```python
from build123d import *

# Parameters (mm, degrees)
SKETCH_1_W          = 76
SKETCH_1_H          = 60
EXTRUDE_1_DEPTH     = 2
EXTRUDE_2_DEPTH     = 3.35
SKETCH_2_W          = 76
SKETCH_2_H          = 60
CUT_EXTRUDE_1_DEPTH = 2.95
SKETCH_3_R          = 1.715
CUT_EXTRUDE_2_DEPTH = 10
SKETCH_5_R          = 1.5
CUT_EXTRUDE_3_DEPTH = 45.193605611
SKETCH_6_R          = 2.5
CUT_EXTRUDE_4_DEPTH = 45.111815616
CUT_EXTRUDE_5_DEPTH = 4
CUT_EXTRUDE_6_DEPTH = 4
CUT_EXTRUDE_7_DEPTH = 4


with BuildPart() as part:
    # 草圖1 → 填料-伸長1 (new body)
    with BuildSketch(Plane.XY):
        Rectangle(SKETCH_1_W, SKETCH_1_H)
        with BuildLine():
            Line((-6.042909564, -9.905650781), (-7.592909564, -12.590329533))
            ThreePointArc((-7.592909564, -12.590329533), (-7.896512744, -12.823292446), (-8.275922266, -12.773342235))
            Line((-8.275922266, -12.773342235), (-10.007973074, -11.773342235))
            ThreePointArc((-10.007973074, -11.773342235), (-10.240935987, -11.469739056), (-10.190985776, -11.090329533))
            Line((-10.190985776, -11.090329533), (-8.640985776, -8.405650781))
            ThreePointArc((-8.640985776, -8.405650781), (-8.337382596, -8.172687868), (-7.957973074, -8.22263808))
            Line((-7.957973074, -8.22263808), (-6.225922266, -9.22263808))
            ThreePointArc((-6.225922266, -9.22263808), (-5.992959353, -9.526241259), (-6.042909564, -9.905650781))
        make_face(mode=Mode.SUBTRACT)
        with BuildLine():
            ThreePointArc((-14.313100093, -9.230040965), (-14.996112795, -9.413053667), (-15.179125497, -8.730040965))
            Line((-15.179125497, -8.730040965), (-13.179125497, -5.26593935))
            ThreePointArc((-13.179125497, -5.26593935), (-12.496112795, -5.082926648), (-12.313100093, -5.76593935))
            Line((-12.313100093, -5.76593935), (-14.313100093, -9.230040965))
        make_face(mode=Mode.SUBTRACT)
        with BuildLine():
            ThreePointArc((11.146484837, -8.780487805), (10.646484837, -8.280487805), (11.146484837, -7.780487805))
            Line((11.146484837, -7.780487805), (15.146484837, -7.780487805))
            ThreePointArc((15.146484837, -7.780487805), (15.646484837, -8.280487805), (15.146484837, -8.780487805))
            Line((15.146484837, -8.780487805), (11.146484837, -8.780487805))
        make_face(mode=Mode.SUBTRACT)
        with BuildLine():
            Line((-5.557090436, 10.186138586), (-7.107090436, 12.870817338))
            ThreePointArc((-7.107090436, 12.870817338), (-7.157040647, 13.250226861), (-6.924077734, 13.55383004))
            Line((-6.924077734, 13.55383004), (-5.192026926, 14.55383004))
            ThreePointArc((-5.192026926, 14.55383004), (-4.812617404, 14.603780251), (-4.509014224, 14.370817338))
            Line((-4.509014224, 14.370817338), (-2.959014224, 11.686138586))
            ThreePointArc((-2.959014224, 11.686138586), (-2.909064013, 11.306729064), (-3.142026926, 11.003125884))
            Line((-3.142026926, 11.003125884), (-4.874077734, 10.003125884))
            ThreePointArc((-4.874077734, 10.003125884), (-5.253487256, 9.953175673), (-5.557090436, 10.186138586))
        make_face(mode=Mode.SUBTRACT)
        with BuildLine():
            Line((1.163100093, 13.546427155), (-0.836899907, 17.01052877))
            ThreePointArc((-0.836899907, 17.01052877), (-0.653887205, 17.693541472), (0.029125497, 17.51052877))
            Line((0.029125497, 17.51052877), (2.029125497, 14.046427155))
            ThreePointArc((2.029125497, 14.046427155), (1.846112795, 13.363414453), (1.163100093, 13.546427155))
        make_face(mode=Mode.SUBTRACT)
    extrude(amount=EXTRUDE_1_DEPTH)

    # 草圖1<3> → 填料-伸長2 (add)
    with BuildSketch(Plane.XY):
        with BuildLine():
            Line((14.696484837, -0.280487805), (11.596484837, -0.280487805))
            ThreePointArc((11.596484837, -0.280487805), (11.242931447, -0.426934414), (11.096484837, -0.780487805))
            Line((11.096484837, -0.780487805), (11.096484837, -2.780487805))
            ThreePointArc((11.096484837, -2.780487805), (11.242931447, -3.134041195), (11.596484837, -3.280487805))
            Line((11.596484837, -3.280487805), (14.696484837, -3.280487805))
            ThreePointArc((14.696484837, -3.280487805), (15.050038228, -3.134041195), (15.196484837, -2.780487805))
            Line((15.196484837, -2.780487805), (15.196484837, -0.780487805))
            ThreePointArc((15.196484837, -0.780487805), (15.050038228, -0.426934414), (14.696484837, -0.280487805))
        make_face()
        with BuildLine():
            Line((-7.592909564, -12.590329533), (-6.042909564, -9.905650781))
            ThreePointArc((-6.042909564, -9.905650781), (-5.992959353, -9.526241259), (-6.225922266, -9.22263808))
            Line((-6.225922266, -9.22263808), (-7.957973074, -8.22263808))
            ThreePointArc((-7.957973074, -8.22263808), (-8.337382596, -8.172687868), (-8.640985776, -8.405650781))
            Line((-8.640985776, -8.405650781), (-10.190985776, -11.090329533))
            ThreePointArc((-10.190985776, -11.090329533), (-10.240935987, -11.469739056), (-10.007973074, -11.773342235))
            Line((-10.007973074, -11.773342235), (-8.275922266, -12.773342235))
            ThreePointArc((-8.275922266, -12.773342235), (-7.896512744, -12.823292446), (-7.592909564, -12.590329533))
        make_face()
        with BuildLine():
            Line((-7.107090436, 12.870817338), (-5.557090436, 10.186138586))
            ThreePointArc((-5.557090436, 10.186138586), (-5.253487256, 9.953175673), (-4.874077734, 10.003125884))
            Line((-4.874077734, 10.003125884), (-3.142026926, 11.003125884))
            ThreePointArc((-3.142026926, 11.003125884), (-2.909064013, 11.306729064), (-2.959014224, 11.686138586))
            Line((-2.959014224, 11.686138586), (-4.509014224, 14.370817338))
            ThreePointArc((-4.509014224, 14.370817338), (-4.812617404, 14.603780251), (-5.192026926, 14.55383004))
            Line((-5.192026926, 14.55383004), (-6.924077734, 13.55383004))
            ThreePointArc((-6.924077734, 13.55383004), (-7.157040647, 13.250226861), (-7.107090436, 12.870817338))
        make_face()
    extrude(amount=EXTRUDE_2_DEPTH)

    # 草圖2 → 除料-伸長1 (cut)
    with BuildSketch(Plane(origin=(0, 0, 0), x_dir=(-1, 0, 0), z_dir=(0, 0, -1))):
        Rectangle(SKETCH_2_W, SKETCH_2_H)
        with BuildLine():
            ThreePointArc((-29.9, 26.904317068), (-33.435533906, 25.439850974), (-34.9, 21.904317068))
            Line((-34.9, 21.904317068), (-34.9, -21.9))
            ThreePointArc((-34.9, -21.9), (-33.435533906, -25.435533906), (-29.9, -26.9))
            Line((-29.9, -26.9), (29.9, -26.9))
            ThreePointArc((29.9, -26.9), (33.435533906, -25.435533906), (34.9, -21.9))
            Line((34.9, -21.9), (34.9, 21.904317068))
            ThreePointArc((34.9, 21.904317068), (33.435533906, 25.439850974), (29.9, 26.904317068))
            Line((29.9, 26.904317068), (-29.9, 26.904317068))
        make_face(mode=Mode.SUBTRACT)
    extrude(amount=-CUT_EXTRUDE_1_DEPTH, mode=Mode.SUBTRACT)

    # 草圖3 → 除料-伸長2 (cut)
    with BuildSketch(Plane(origin=(0, 0, 0), x_dir=(-1, 0, 0), z_dir=(0, 0, -1))):
        Circle(SKETCH_3_R)
    extrude(amount=-CUT_EXTRUDE_2_DEPTH, mode=Mode.SUBTRACT)

    # 草圖4 → 除料-旋轉1 (revolve, cut)
    with BuildSketch(Plane(origin=(0, 0, 0), x_dir=(1, 0, 0), z_dir=(0, 1, 0)), mode=Mode.PRIVATE) as cut_revolve_1_sk:
        Polygon((0, -2), (11, -2), (13, 0), (0, 0), align=None)
    revolve(cut_revolve_1_sk.sketch.rotate(Axis((0, 0, -2.897060396), (0, 0, 1)), 180), axis=Axis((0, 0, -2.897060396), (0, 0, 1)), mode=Mode.SUBTRACT)

    # 草圖5 → 除料-伸長3 (cut, through all)
    with BuildSketch(Plane.XY):
        with Locations((32.4, 17.904317068)):
            Circle(SKETCH_5_R)
        with Locations((-32.4, 19.404317068)):
            Circle(SKETCH_5_R)
        with Locations(Location((-32.4, -19.4, 0), (0, 0, 180))):
            Circle(SKETCH_5_R)
        with Locations((32.4, -19.4)):
            Circle(SKETCH_5_R)
    extrude(amount=CUT_EXTRUDE_3_DEPTH, mode=Mode.SUBTRACT)

    # 草圖6 → 除料-伸長4 (cut, through all)
    with BuildSketch(Plane.XY.offset(2)):
        with Locations((-21.9, 16.904317068)):
            Circle(SKETCH_6_R)
        with Locations(Location((21.9, 16.904317068, 0), (0, 0, 180))):
            Circle(SKETCH_6_R)
        with Locations((-21.9, -19.4)):
            Circle(SKETCH_6_R)
    extrude(amount=-CUT_EXTRUDE_4_DEPTH, mode=Mode.SUBTRACT)

    # 草圖7 → 除料-伸長5 (cut)
    with BuildSketch(Plane.ZY.offset(-11.146484837)):
        Polygon((2, -8.780487805), (2, -11.780487805), (0, -13.780487805), (0, -8.780487805), align=None)
    extrude(amount=-CUT_EXTRUDE_5_DEPTH, mode=Mode.SUBTRACT)

    # 草圖8 → 除料-伸長6 (cut)
    with BuildSketch(Plane(origin=(-5.575, -9.656183252, 0), x_dir=(0.8660254037844398, -0.499999999999998, 0), z_dir=(0.49999999999999806, 0.8660254037844399, 0))):
        Polygon((-8.780487805, -2), (-8.780487805, 0), (-13.780487805, 0), (-11.780487805, -2), align=None)
    extrude(amount=-CUT_EXTRUDE_6_DEPTH, mode=Mode.SUBTRACT)

    # 草圖9 → 除料-伸長7 (cut)
    with BuildSketch(Plane(origin=(-5.575, 9.656183252, 0), x_dir=(-0.8660254037844397, -0.49999999999999806, 0), z_dir=(0.49999999999999806, -0.8660254037844397, 0))):
        Polygon((-8.780487805, -2), (-8.780487805, 0), (-13.780487805, 0), (-11.780487805, -2), align=None)
    extrude(amount=-CUT_EXTRUDE_7_DEPTH, mode=Mode.SUBTRACT)


solid = part.part
```
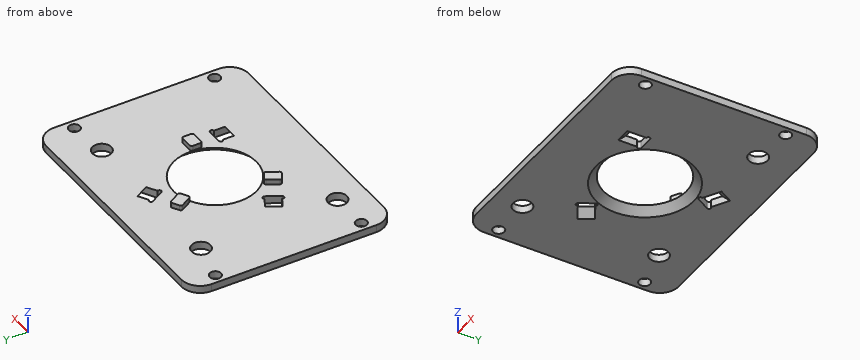
Verification items for the finished model (mm, model axes). Round coordinates to 2 decimals unless told otherwise and drop trailing zeros. Write each loop counter-clockwise with the first axis right and the second up, starting at its lowest first coordinate (ties: lowest second). Pieces come first, ordered by that corner, then holes. Notation, with made-up numbers: (87.25, 73) -> (112.25, 73) arc R20 ccw to (112.25, 108) -> close; hole circle Ø1 at (65.5, 64.25). An arc over 180 degrees is marked (long way). Write each question's results on one line, items separated by ' | '.
Q1. Go/stop test with flat-tipped pins: pin 1 Ø0.7 at (y, z) = (-1.5, 2.5) entering from +X; pin 2 Ø5 at (x, y) = (1.5, 8.5) entering from +Z; pin 3 Ø0.7 at (x, z) = (13.5, 3) entering from +Y. Record where each tip stops, or that it passes through.
Derived:
pin 1: stops at x = 15.2 | pin 2: stops at z = 2 | pin 3: stops at y = -0.28
Q2. Sectioned sample at B-B, the plane x = -21.9. Record the boundary of the cut face in (y, z).
Derived:
outline: (-26.9, 0) -> (-21.9, 0) -> (-21.9, 2) -> (-26.9, 2) -> close; (-16.9, 0) -> (14.4, 0) -> (14.4, 2) -> (-16.9, 2) -> close; (19.4, 0) -> (26.9, 0) -> (26.9, 2) -> (19.4, 2) -> close
Q3. Sectioned sample at C-C, the plane x = 23. Record the boundary of the cut face in (y, z).
Derived:
outline: (-26.9, 0) -> (14.66, 0) -> (14.66, 2) -> (-26.9, 2) -> close; (19.15, 0) -> (26.9, 0) -> (26.9, 2) -> (19.15, 2) -> close
Q4. Thickness scan on probe 1 along Y at (x, z) = (-32.4, 1.2); probe 2 along Y at (x, z) = (32.4, 1.55); probe 3 along Z at (x, y) = (7, -13.5). Record the ranges inside material, lowest first.
Derived:
probe 1: y = -26.23 to -20.9, -17.9 to 17.9, 20.9 to 26.23 | probe 2: y = -26.23 to -20.9, -17.9 to 16.4, 19.4 to 26.23 | probe 3: z = 0 to 2
Q5. Sectioned sample at D-D, the plane x = -32.4. Record the boundary of the cut face in (y, z).
Derived:
outline: (-26.23, 0) -> (-20.9, 0) -> (-20.9, 2) -> (-26.23, 2) -> close; (-17.9, 0) -> (17.9, 0) -> (17.9, 2) -> (-17.9, 2) -> close; (20.9, 0) -> (26.23, 0) -> (26.23, 2) -> (20.9, 2) -> close
Q6. Sectioned sample at A-A, the plane z = 2.6. Record the boundary of the cut face in (x, y), and give its area (3 significant figures).
Derived:
outline: (-10.19, -11.09) arc R0.5 ccw to (-10.01, -11.77) -> (-8.28, -12.77) arc R0.5 ccw to (-7.59, -12.59) -> (-6.04, -9.91) arc R0.5 ccw to (-6.23, -9.22) -> (-7.96, -8.22) arc R0.5 ccw to (-8.64, -8.41) -> close; (-7.11, 12.87) -> (-5.56, 10.19) arc R0.5 ccw to (-4.87, 10) -> (-3.14, 11) arc R0.5 ccw to (-2.96, 11.69) -> (-4.51, 14.37) arc R0.5 ccw to (-5.19, 14.55) -> (-6.92, 13.55) arc R0.5 ccw to start; (11.1, -2.78) arc R0.5 ccw to (11.6, -3.28) -> (14.7, -3.28) arc R0.5 ccw to (15.2, -2.78) -> (15.2, -0.78) arc R0.5 ccw to (14.7, -0.28) -> (11.6, -0.28) arc R0.5 ccw to (11.1, -0.78) -> close | area: 36.3 mm²
